```python
from build123d import *

# Parameters (mm, degrees)
F1_DEPTH = 42.5
F3_DEPTH = 174
F4_R     = 12.5
F5_DEPTH = 266
F6_W     = 40
F6_H     = 260
F7_DEPTH = 40


with BuildPart() as f1:
    # F0 (on Right) → F1 (new body, symmetric)
    with BuildSketch(Plane.YZ):
        with BuildLine():
            ThreePointArc((61.934647, 39.548864), (71.990491, 30.564401), (64.190836, 19.564131))
            Line((64.190836, 19.564131), (52.245142, 19.564131))
            Line((52.245142, 19.564131), (-156.829834, 19.564131))
            Line((-156.829834, 19.564131), (-156.829834, -25.435869))
            Line((-156.829834, -25.435869), (113.170166, -25.435869))
            Line((113.170166, -25.435869), (113.170166, 19.564131))
            ThreePointArc((113.170166, 19.564131), (97.724143, 54.982764), (61.934647, 69.548864))
            Line((61.934647, 69.548864), (36.934647, 69.548864))
            Line((36.934647, 69.548864), (36.934647, 39.548864))
            Line((36.934647, 39.548864), (61.934647, 39.548864))
        make_face()
    extrude(amount=F1_DEPTH, both=True)

    # F2 (on Front) → F3 (cut, symmetric)
    with BuildSketch(Plane.XZ):
        with BuildLine():
            Line((23.624079, 19.918991), (23.624079, -36.902788))
            Line((23.624079, -36.902788), (-26.375921, -36.902788))
            Line((-26.375921, -36.902788), (-26.375921, 19.918991))
            ThreePointArc((-26.375921, 19.918991), (-30.233422, 35.78282), (-44.975936, 42.797067))
            Line((-44.975936, 42.797067), (-64.052075, -61.106175))
            Line((-64.052075, -61.106175), (44.571461, -67.325629))
            Line((44.571461, -67.325629), (64.148389, 37.735406))
            Line((64.148389, 37.735406), (42.224093, 42.797067))
            ThreePointArc((42.224093, 42.797067), (27.481579, 35.78282), (23.624079, 19.918991))
        make_face()
    extrude(amount=F3_DEPTH, both=True, mode=Mode.SUBTRACT)

    # F4 (on Front) → F5 (cut, symmetric)
    with BuildSketch(Plane.XZ):
        with Locations((-1.375921, -2.935869)):
            Circle(F4_R)
    extrude(amount=F5_DEPTH, both=True, mode=Mode.SUBTRACT)

    # F6 (on face) → F7 (cut)
    with BuildSketch(Plane(origin=(0, 0, -25.435869), x_dir=(1, 0, 0), z_dir=(0, 0, -1))):
        with Locations((-1.719187, 21.451403)):
            Rectangle(F6_W, F6_H)
    extrude(amount=-F7_DEPTH, mode=Mode.SUBTRACT)


solid = f1.part
```
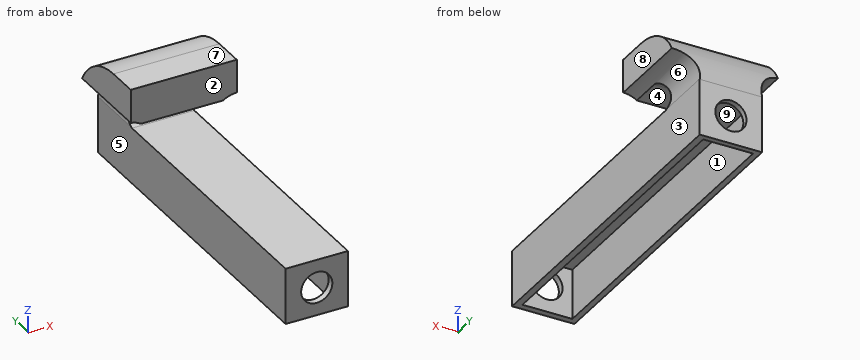
Input: part model. Units: mm. Frame: model coordinates. Face numbers are marked on the shaded views. A direction names the side the tool comes from. Give positions to 0.01 mm unless a question says otherwise; leave off trailing zeros. Order: outer loops, then holes, each group sorted by start corner. A loop starts at its lowest first (then second) coordinate and runs counter-clockwise, first axis right, second up. Notation, with made-up numbers: M -12,-15.75 L 17,-15.75 A14 cw 17,-8.75 Z; hole C -6.5,44 d9. An arc over 180 degrees is marked long. One line per question, with ' | ' between items. Start each with the question number.
1. Section query D-D (z = 2.5). Return the cut outline in (x, y), and give its area (3 significant figures).
2. Access query for the marked faces 1, 2, 3, 4 and 5. Directions: +Z, -Z, +X, -X, +Y, -Y. A direction counts if a zero-diameter tool reaches every point of the face in a straight line with its end or side. Return the directions, or none.
3. Section query C-C (x = -18.5). Return the cut outline in (y, z).
4. Pull-direction query (Z, two-part tool) for the marked faces 6, 7, 8 and 9; classes: released by +Z, released by -Z, zero draft, split by the parting line, or undercut.
5. Section query A-A (y = -76.5). Return the cut outline in (x, z).
6. First-contact query: pin 1 Ø8 at (x, z) = (26.5, 57) entering from +Y; pin 2 Ø6 at (x, z) = (-10.5, 32) entering from -Y; pin 3 Ø1 at (x, z) = (30, 49.5) entering from -Y; pin 4 Ø20 at (x, z) = (-1.38, -2.94) entering from +Y. Flat tips, straight axial feed; report the tip coordinate or a pass-through.
7. Material intervals for probe 1 along X at (y, z) = (99, 8.5); probe 2 along Z at (x, y) = (9, -19); probe 3 along Y at (x, z) = (0.5, -21), sorted ascending. Write a range as [from, to].
8. Section query B-B (x = -7.5). Return the cut outline in (y, z), and give its area (3 significant figures).
Here are the results:
1) outline: M -26.38,-156.83 L -12.63,-156.83 L -12.63,-151.45 L -21.72,-151.45 L -21.72,108.55 L -12.63,108.55 L -12.63,113.17 L -26.38,113.17 Z; M 9.88,-156.83 L 23.62,-156.83 L 23.62,113.17 L 9.88,113.17 L 9.88,108.55 L 18.28,108.55 L 18.28,-151.45 L 9.88,-151.45 Z | area: 2,870 mm²
2) face 1: -Z | face 2: +Z, +X, -X, -Y | face 3: -Z, +X, +Y, -Y | face 4: +X, -X, -Y | face 5: -Z, -X, +Y, -Y
3) outline: M -156.83,-25.44 L -151.45,-25.44 L -151.45,14.56 L 108.55,14.56 L 108.55,-25.44 L 113.17,-25.44 L 113.17,19.56 A51.25 ccw 61.93,69.55 L 36.93,69.55 L 36.93,39.55 L 61.93,39.55 A10.12 cw 64.19,19.56 L -156.83,19.56 Z
4) face 6: undercut | face 7: released by +Z | face 8: zero draft | face 9: released by -Z
5) outline: M -26.38,-25.44 L -21.72,-25.44 L -21.72,14.56 L 18.28,14.56 L 18.28,-25.44 L 23.62,-25.44 L 23.62,19.56 L -26.38,19.56 Z
6) pin 1: y = 99.65 | pin 2: y = 70.38 | pin 3: y = 36.93 | pin 4: through
7) probe 1: [-26.38, -21.72], [18.28, 23.62] | probe 2: [14.56, 19.56] | probe 3: [-156.83, -151.45], [108.55, 113.17]
8) outline: M -156.83,-25.44 L -151.45,-25.44 L -151.45,-13.83 L -156.83,-13.83 Z; M -156.83,7.96 L -151.45,7.96 L -151.45,14.56 L 108.55,14.56 L 108.55,7.96 L 113.17,7.96 L 113.17,19.56 A51.25 ccw 61.93,69.55 L 36.93,69.55 L 36.93,39.55 L 61.93,39.55 A10.12 cw 64.19,19.56 L -156.83,19.56 Z; M 108.55,-25.44 L 113.17,-25.44 L 113.17,-13.83 L 108.55,-13.83 Z | area: 4,120 mm²
